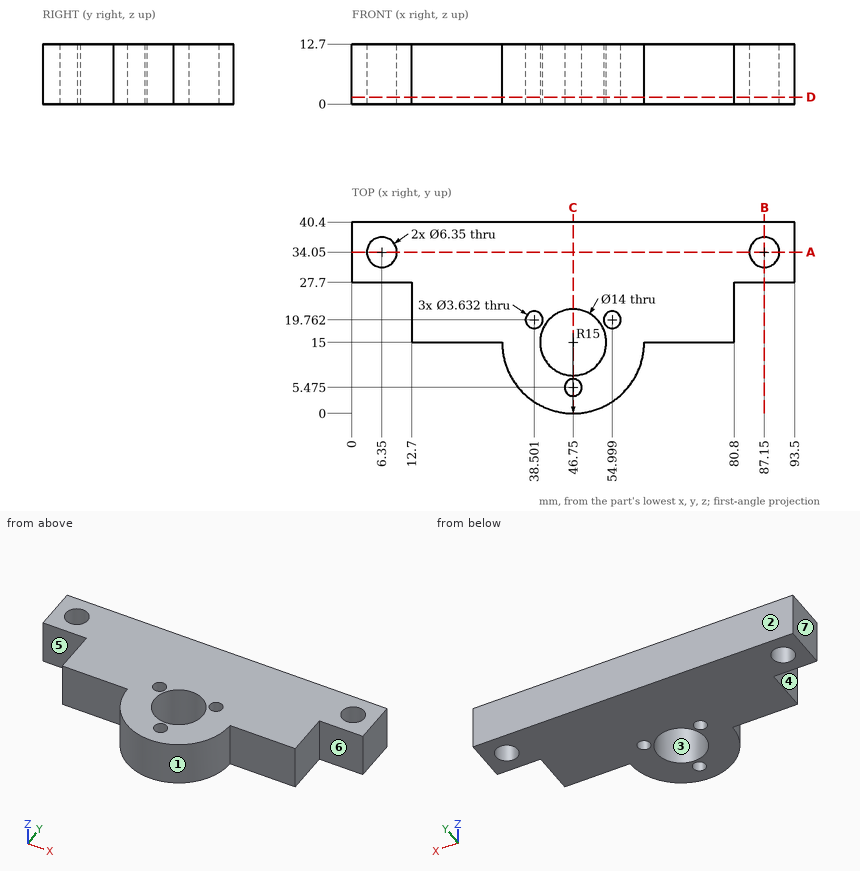
For this review, use the dimensioned drawing (mm, ordinates from the lowest corner) and the shaded views. A direction names the side the tool comes from. Coordinates: 2 decimals unless noted, no trailing zeros. Order: outer loops, then holes, each group sorted by start corner. A loop starts at its lowest first (then second) coordinate and runs counter-clockwise, first axis right, second up. Notation, with made-up numbers: M -25.75,43.25 L -20.75,43.25 A13 ccw -20.75,48.25 Z; hole C -33.5,-11.75 d4. An arc over 180 degrees is marked long. Answer as a JSON object with one key per item and string values. Group by question number.
1) Tool access review of the marked faces 5, 6 and 7: name each direction out of +Z, -Z, +X, -X, +Y, -Y from which nothing blocks a thin tool from reaching the whole face with its end or side.
2) Add section B-B, the plane x = 87.15. Write out the cut boundary in (y, z) (1 decimal).
3) Mouldability with a two-part tool opening along Y and no side actions: class the marked faces 1, 2, 3 and 4 as pulls with the +Y half, pulls with the -Y half, needs draft (parallel to the pull), parting line crosses it, or undercut.
4) Wall thickness on L1, parallel to Y at x = 46.75, z = 6.75; L2, parallel to Y at x = 6.35, z = 3.5 (1 decimal); L3, parallel to X at y = 32.5, z = 8.5: over which ranges is each line inside the solid? List them lowest first.
5) Add section C-C, the plane x = 46.75. Write out the cut boundary in (y, z), then the cut area to 3 significant figures.
6) Add section A-A, the plane y = 34.05. Write out the cut boundary in (x, z) (1 decimal), then the cut area to 3 significant figures.
7) Add section D-D, the plane z = 1.5. Count the separate pieces of the cut face and the enclosed holes in it, then the cut area to 3 significant figures.
8) For pin 1 (1.5 mm diameter, centred on y = 9.5, z = 10, fed in from -X); pin 2 (6.5 mm diameter, centred on y = 23.5, z = 8, fed in from +X); pin 3 (3 mm diameter, centred on x = 43.5, z = 5.5, fed in from -Y), all flat-tipped, find the tip position at first contact; note any pin that passes through.
Computed values:
{
 "1": {"face 5": "+Z, -Z, -X, -Y", "face 6": "+Z, -Z, +X, -Y", "face 7": "+Z, -Z, -X, +Y, -Y"},
 "2": {"outline": "M 27.7,0 L 30.9,0 L 30.9,12.7 L 27.7,12.7 Z; M 37.2,0 L 40.4,0 L 40.4,12.7 L 37.2,12.7 Z"},
 "3": {"face 1": "pulls with the -Y half", "face 2": "pulls with the +Y half", "face 3": "undercut", "face 4": "needs draft"},
 "4": {"L1": "y = 0 to 3.66, 7.29 to 8, 22 to 40.4", "L2": "y = 27.7 to 30.9, 37.2 to 40.4", "L3": "x = 0 to 3.58, 9.12 to 84.38, 89.92 to 93.5"},
 "5": {"outline": "M 0,0 L 3.66,0 L 3.66,12.7 L 0,12.7 Z; M 7.29,0 L 8,0 L 8,12.7 L 7.29,12.7 Z; M 22,0 L 40.4,0 L 40.4,12.7 L 22,12.7 Z", "area": "289 mm^2"},
 "6": {"outline": "M 0,0 L 3.2,0 L 3.2,12.7 L 0,12.7 Z; M 9.5,0 L 84,0 L 84,12.7 L 9.5,12.7 Z; M 90.3,0 L 93.5,0 L 93.5,12.7 L 90.3,12.7 Z", "area": "1,030 mm^2"},
 "7": {"separate pieces": "1", "enclosed holes": "6", "area": "2,160 mm^2"},
 "8": {"pin 1": "stops at x = 32.52", "pin 2": "stops at x = 80.8", "pin 3": "stops at y = 0.1"}
}
